from build123d import *

# Parameters (mm, degrees)
SKETCH1_W           = 2.5
SKETCH1_H           = 24
SKETCH1_W_2         = 12
SKETCH1_H_2         = 2.5
BOSS_EXTRUDE1_DEPTH = 10
CUT_EXTRUDE1_DEPTH  = 10
CUT_EXTRUDE2_DEPTH  = 0.5
SKETCH5_W           = 3
SKETCH5_H           = 24
SKETCH5_W_2         = 9
SKETCH5_H_2         = 2.5
BOSS_EXTRUDE2_DEPTH = 2
CHAMFER1_SIZE       = 0.5


with BuildPart() as part:
    # Sketch1 → Boss-Extrude1 (new body)
    with BuildSketch(Plane(origin=(0, 0, 0), x_dir=(0, 0, -1), z_dir=(1, 0, 0))):
        with Locations((1.25, 14.5)):
            Rectangle(SKETCH1_W, SKETCH1_H)
        with Locations((8.5, 1.25)):
            Rectangle(SKETCH1_W_2, SKETCH1_H_2)
        with Locations((1.25, 1.25)):
            Rectangle(SKETCH1_W, SKETCH1_H_2)
    extrude(amount=BOSS_EXTRUDE1_DEPTH)

    # Sketch2 → Cut-Extrude1 (cut)
    with BuildSketch(Plane.XY):
        with BuildLine():
            ThreePointArc((6.7, 21.5), (6.202081528, 22.702081528), (5, 23.2))
            Line((5, 23.2), (5, 19.8))
            ThreePointArc((5, 19.8), (6.202081528, 20.297918472), (6.7, 21.5))
        make_face()
        with BuildLine():
            Line((5, 19.8), (5, 23.2))
            ThreePointArc((5, 23.2), (3.3, 21.5), (5, 19.8))
        make_face()
    extrude(amount=-CUT_EXTRUDE1_DEPTH, mode=Mode.SUBTRACT)

    # Sketch4 → Cut-Extrude2 (cut)
    with BuildSketch(Plane.XY):
        Polygon((5, 24.790896534), (2.15, 23.145448267), (2.15, 19.854551733), (5, 18.209103466), (7.85, 19.854551733), (7.85, 23.145448267), align=None)
    extrude(amount=-CUT_EXTRUDE2_DEPTH, mode=Mode.SUBTRACT)

    # Sketch5 → Boss-Extrude2 (add)
    with BuildSketch(Plane.ZY):
        with Locations((-4, 14.5)):
            Rectangle(SKETCH5_W, SKETCH5_H)
        Polygon((-5.5, 0), (0, 0), (0, 26.5), (-2.5, 26.5), (-2.5, 2.5), (-5.5, 2.5), align=None)
        with Locations((-10, 1.25)):
            Rectangle(SKETCH5_W_2, SKETCH5_H_2)
    extrude(amount=BOSS_EXTRUDE2_DEPTH)

    # Chamfer1
    chamfer1_edges = [part.edges().sort_by_distance(p)[0] for p in [
        (10, 0, -7.25),
        (4, 26.5, 0),
        (5, 26.5, -2.5),
        (4, 2.5, -14.5),
        (4, 0, -14.5),
        (4, 0, 0),
        (10, 1.25, -14.5),
        (10, 2.5, -8.5),
        (10, 14.5, -2.5),
        (10, 26.5, -1.25),
        (10, 13.25, 0),
        (-2, 14.5, -5.5),
        (-1, 26.5, -5.5),
        (0, 26.5, -4),
        (-2, 2.5, -10),
        (-2, 1.25, -14.5),
        (-2, 0, -7.25),
        (-2, 13.25, 0),
        (-2, 26.5, -2.75),
    ]]
    chamfer(chamfer1_edges, length=CHAMFER1_SIZE)


solid = part.part
Build history of the part. All positions in model axes, mm. A direction names the side the tool comes from. Round coordinates to 2 decimals unless told otherwise and drop trailing zeros. Write each loop counter-clockwise with the first axis right and the second up, starting at its lowest first coordinate (ties: lowest second). Pieces come first, ordered by that corner, then holes. Notation, with made-up numbers: M 88,75.5 L 128,75.5 A29 ccw 128,103.5 Z; hole C 37,58 d9. An arc over 180 degrees is marked long. Answer as a JSON object with one key per item and string values. Group by question number.
(1) Drill centre lines: L1, parallel to X at y = 18.5, z = -3; L2, parallel to Z at x = 5.75, y = 8; L3, parallel to Y at x = 6.5, z = -13.75. Where is each one in solid material? Low to high.
(2) Cut at D-D (z = -3.5). Give the cut face in (x, y).
(3) Cut at B-B (y = 11.25). Give the cut face in (x, z), and give its area (3 significant figures).
(4) Which spindle directions (+Z, -Z, +X, -X, +Y, -Y) get a long thin tool onto all of the face, cutting with end or side? Do faces 4 (the flat face through (0, 14, -4)), 5 (the flat face through (6.44, 23.96, -0.25)), 6 (the flat face through (-1, 14, -5.5)). Say none if no direction does.
(5) Cut at A-A (x = 0.75). Give the cut face in (y, z), and give its area (3 significant figures).
(6) Cut at C-C (z = -12). Give the cut face in (x, y).
(7) Mould opens along X. For faces 1 (the flat face through (10, 9.5, -1.7)), 2 (the flat face through (3.56, 19.04, -0.25)), 3 (the flat face through (4, 13, 0)) say: pulls with the +X half, pulls with the -X half, needs draft (parallel to the pull), parting line crosses it, or undercut.
(8) Flat gauge pins, fed straight in: pin 1 (5 mm diameter, centred on x = 0.5, y = 10.5, fed in from -Z); pin 2 (0.9 mm diameter, centred on y = 19.5, z = -4.5, fed in from +X); pin 3 (5.5 mm diameter, centred on x = 1.5, z = -8, fed in from +Y). Where does each tip first touch, or does it go through?
Responses:
{
 "1": {"L1": "x = -2 to 0", "L2": "z = -2.5 to 0", "L3": "y = 0 to 2.5"},
 "2": {"outline": "M -2,0.5 L -1.5,0 L 9.5,0 L 10,0.5 L 10,2 L 9.5,2.5 L 0,2.5 L 0,26 L -0.5,26.5 L -1.5,26.5 L -2,26 Z"},
 "3": {"outline": "M -2,-5 L -1.5,-5.5 L 0,-5.5 L 0,-2.5 L 9.5,-2.5 L 10,-2 L 10,-0.5 L 9.5,0 L -1.5,0 L -2,-0.5 Z", "area": "35.5 mm2"},
 "4": {"face 4": "-Z, +X, +Y", "face 5": "+Z", "face 6": "-Z, +X, -X, +Y"},
 "5": {"outline": "M 0,-14 L 0.5,-14.5 L 2,-14.5 L 2.5,-14 L 2.5,-2.5 L 26,-2.5 L 26.5,-2 L 26.5,-0.5 L 26,0 L 0.5,0 L 0,-0.5 Z", "area": "95.6 mm2"},
 "6": {"outline": "M -2,0.5 L -1.5,0 L 9.5,0 L 10,0.5 L 10,2 L 9.5,2.5 L -1.5,2.5 L -2,2 Z"},
 "7": {"face 1": "pulls with the +X half", "face 2": "undercut", "face 3": "needs draft"},
 "8": {"pin 1": "stops at z = -5.5", "pin 2": "stops at x = 0", "pin 3": "stops at y = 2.5"}
}
